Autodesk Inventor part; units mm, degrees
ref_plane "YZ Plane" through (0, 0, 0) normal (1, 0, 0) x (0, 1, 0)
ref_plane "XZ Plane" through (0, 0, 0) normal (0, 1, 0) x (-1, 0, 0)
ref_plane "XY Plane" through (0, 0, 0) normal (0, 0, 1) x (1, 0, 0)
sketch "Sketch1" plane through (0, 0, 0) normal (0, 0, 1) x (1, 0, 0)
  line L0 (-30, 7.5) -> (30, 7.5)
  line L1 (30, 7.5) -> (30, -7.5)
  line L2 (30, -7.5) -> (-30, -7.5)
  line L3 (-30, -7.5) -> (-30, 7.5)
  line L4 (-42, 0) -> (42, 0)
  line L5 (0, -10.5) -> (0, 10.5)
  line L6 (-15, 2.5) -> (15, 2.5)
  line L7 (15, 2.5) -> (15, -2.5)
  line L8 (15, -2.5) -> (-15, -2.5)
  line L9 (-15, -2.5) -> (-15, 2.5)
  point P0 (0, 0)
  dimension "d0" = 30
  dimension "d1" = 5
  dimension "d2" = 60
  dimension "d3" = 15
extrude "Extrusion1" add sketch "Sketch1" along normal blind 1.2 contours L0 L5 L6 L9 L4 L3 | L0 L1 L4 L7 L6 L5 | L4 L9 L8 L5 L2 L3 | L1 L2 L5 L8 L7 L4
sketch "Sketch2" plane through (0, 0, 1.2) normal (0, 0, 1) x (1, 0, 0)
  line L0 (0, -10.5) -> (0, 10.5)
  line L1 (-42, 0) -> (42, 0)
  line L2 (-21.75, 3.75) -> (21.75, 3.75)
  line L3 (21.75, 3.75) -> (21.75, -3.75)
  line L4 (21.75, -3.75) -> (-21.75, -3.75)
  line L5 (-21.75, -3.75) -> (-21.75, 3.75)
  line L6 (-15, -2.5) -> (-15, 2.5)
  line L7 (-15, 2.5) -> (15, 2.5)
  line L8 (15, -2.5) -> (-15, -2.5)
  line L9 (15, 2.5) -> (15, -2.5)
  point P0 (0, 0)
  dimension "d6" = 43.5
  dimension "d7" = 7.5
extrude "Extrusion2" add sketch "Sketch2" along normal blind 3 contours L4 L5 L1 L6 L8 L0 | L0 L8 L9 L1 L3 L4 | L1 L9 L7 L0 L2 L3 | L5 L2 L0 L7 L6 L1
Source: CAD feature listing. Evaluate the final solid. Frame: model axes, mm. A direction names the side the tool comes from. Give positions to 0.01 mm unless a question says otherwise; leave off trailing zeros. Loops run counter-clockwise (first coordinate to the right, second up) from the corner with the lowest first, then second, coordinate; pieces in that order, holes last. Notation, with made-up numbers: (-17, 44) - (29, 44) arc R15 cw to (29, 57) - close; hole circle Ø9 at (-24.5, -22). An arc over 180 degrees is marked (long way). Use CSV: the item, a comma, the result in double quotes. Start each with the question number.
1. Section D-D (x = 17.5). Output: boundary loops of the cut face in (y, z), then the cut area to 3 significant figures.
2. Pin query (flat end, axial travel): pin 1 (1.5 mm diameter, centred on y = -0.5, z = 3, fed in from +X); pin 2 (4 mm diameter, centred on x = -24, y = 1, fed in from +Z); pin 3 (2.5 mm diameter, centred on x = 4, z = 2.5, fed in from +Y). Return the tip coordinate at first contact, or that it passes through.
3. Section B-B (z = 3.1). Output: boundary loops of the cut face in (x, y), then the cut area to 3 significant figures.
4. Section C-C (y = 1.5). Output: boundary loops of the cut face in (x, z).
5. Ray query, L1, parallel to X at y = 0.75, z = 0.9; L2, parallel to Y at x = -3, z = 2.45; L3, parallel to X at y = 1.5, z = 4. Return the intervals inside material, ascending.
6. Reachability of faces 1 (the flat face through (0, 3.75, 3)), 2 (the flat face through (0, -2.5, 2)), 3 (the flat face through (-21.75, 0, 3)), 4 (the flat face through (0, -3.75, 3)) from +Z, -Z, +X, -X, +Y, -Y: full face, straight path, thin tool, end or side. Return the list, or none.
7. Draft query along X for faces 5 (the flat face through (-15, 0, 2)), 6 (the flat face through (0, -7.5, 1)), 7 (the flat face through (-30, 0, 1)). Return one class per face: +X half, -X half, draft (parallel to the pull), parting line (faces both ways), or undercut.
8. Section A-A (x = 4.5). Output: boundary loops of the cut face in (y, z), then the cut area to 3 significant figures.
Response:
1,outline,"(-7.5, 0) - (7.5, 0) - (7.5, 1.2) - (3.75, 1.2) - (3.75, 4.2) - (-3.75, 4.2) - (-3.75, 1.2) - (-7.5, 1.2) - close"
1,area,"40.5 mm²"
2,pin 1,"x = 21.75"
2,pin 2,"z = 1.2"
2,pin 3,"y = 3.75"
3,outline,"(-21.75, -3.75) - (21.75, -3.75) - (21.75, 3.75) - (-21.75, 3.75) - close; hole (-15, -2.5) - (15, -2.5) - (15, 2.5) - (-15, 2.5) - close"
3,area,"176 mm²"
4,outline,"(-30, 0) - (-15, 0) - (-15, 4.2) - (-21.75, 4.2) - (-21.75, 1.2) - (-30, 1.2) - close; (15, 0) - (30, 0) - (30, 1.2) - (21.75, 1.2) - (21.75, 4.2) - (15, 4.2) - close"
5,L1,"-30 to -15, 15 to 30"
5,L2,"-3.75 to -2.5, 2.5 to 3.75"
5,L3,"-21.75 to -15, 15 to 21.75"
6,face 1,"+Z, +X, -X, +Y"
6,face 2,"+Z, -Z"
6,face 3,"+Z, -X, +Y, -Y"
6,face 4,"+Z, +X, -X, -Y"
7,face 5,"undercut"
7,face 6,"draft"
7,face 7,"-X half"
8,outline,"(-7.5, 0) - (-2.5, 0) - (-2.5, 4.2) - (-3.75, 4.2) - (-3.75, 1.2) - (-7.5, 1.2) - close; (2.5, 0) - (7.5, 0) - (7.5, 1.2) - (3.75, 1.2) - (3.75, 4.2) - (2.5, 4.2) - close"
8,area,"19.5 mm²"
